from build123d import *

# Parameters (mm, degrees)
BOSS_EXTRUDE1_DEPTH              = 3.175
F_6_CLEARANCE_HOLE1_D            = 4.3053
F_6_CLEARANCE_HOLE2_D            = 4.3053
F_9_64_0_14063_DIAMETER_HOLE1_D  = 3.572002
F_15_32_0_46875_DIAMETER_HOLE1_D = 11.90625
F_1_2_0_5_DIAMETER_HOLE1_D       = 12.7
CUT_EXTRUDE1_REACH               = 5.175
SKETCH12_W                       = 9.525
SKETCH12_H                       = 31.75
FILLET1_R                        = 9.525


with BuildPart() as part:
    # Sketch1 → Boss-Extrude1 (new body)
    with BuildSketch(Plane.XY):
        with BuildLine():
            Line((-29.21, 1.5875), (-29.21, 0))
            Line((-29.21, 0), (0, 0))
            Line((0, 0), (0, 165.1))
            Line((0, 165.1), (-25.4, 165.1))
            Line((-25.4, 165.1), (-25.4, 138.1125))
            ThreePointArc((-25.4, 138.1125), (-26.794903955, 134.744903955), (-30.1625, 133.35))
            Line((-30.1625, 133.35), (-53.848, 133.35))
            Line((-53.848, 133.35), (-59.411809524, 6.35))
            Line((-59.411809524, 6.35), (-33.9725, 6.35))
            ThreePointArc((-33.9725, 6.35), (-30.604903955, 4.955096045), (-29.21, 1.5875))
        make_face()
    extrude(amount=-BOSS_EXTRUDE1_DEPTH)

    # #6 Clearance Hole1 (through all)
    with Locations(Plane.XY):
        with Locations((-47.625, 128.5875), (-6.35, 149.86), (-50.546, 16.51), (-6.35, 16.51)):
            Hole(F_6_CLEARANCE_HOLE1_D / 2)

    # #6 Clearance Hole2 (through all)
    with Locations(Plane.XY):
        with Locations((-43.18, 37.084), (-20.32, 120.65)):
            Hole(F_6_CLEARANCE_HOLE2_D / 2)

    # 9/64 (0.14063) Diameter Hole1 (through all)
    with Locations(Plane.XY):
        with Locations((-38.1, 98.425), (-36.5125, 30.1625)):
            Hole(F_9_64_0_14063_DIAMETER_HOLE1_D / 2)

    # 15/32 (0.46875) Diameter Hole1 (through all)
    with Locations(Plane.XY):
        with Locations((-11.684, 88.9)):
            Hole(F_15_32_0_46875_DIAMETER_HOLE1_D / 2)

    # 1/2 (0.5) Diameter Hole1 (through all)
    with Locations(Plane.XY):
        with Locations((-38.1, 88.9), (-26.9875, 30.1625)):
            Hole(F_1_2_0_5_DIAMETER_HOLE1_D / 2)

    # Sketch12 → Cut-Extrude1 (cut, up to next)
    with BuildSketch(Plane.XY, mode=Mode.PRIVATE) as cut_extrude1_sk1:
        with Locations((-25.4, 149.225)):
            Rectangle(SKETCH12_W, SKETCH12_H)
    cut_extrude1_tool1 = extrude(cut_extrude1_sk1.sketch, amount=-CUT_EXTRUDE1_REACH, mode=Mode.PRIVATE) & part.part
    add(cut_extrude1_tool1.solids().sort_by_distance((-25.4, 149.225, 0))[0], mode=Mode.SUBTRACT)

    # Fillet1
    fillet1_edges = [part.edges().sort_by_distance(p)[0] for p in [
        (-20.6375, 133.35, -1.5875),
    ]]
    fillet(fillet1_edges, radius=FILLET1_R)


solid = part.part
Design review of the part built by this model. Coordinates are the model's own, in mm. A direction names the side the tool comes from. Round coordinates to 2 decimals unless told otherwise and drop trailing zeros. Loops run counter-clockwise (first coordinate to the right, second up) from the corner with the lowest first, then second, coordinate; pieces in that order, holes last. Notation, with made-up numbers: (32, 55.5) -> (51, 55.5) arc R29 cw to (51, 77.5) -> close; hole circle Ø10 at (24, 25). An arc over 180 degrees is marked (long way). Use one line per item in the form item = value. Start each with the question number.
Q1. We need section C-C on y = 16.51. Give the boundary of the cut face in (x, z) (3 decimals).
Q2. Draft analysis for pull direction Y (two halves, no side actions). For faces 1 (the face through (-35.196, 31.37, -1.61)), 2 (the face through (-37.713, 96.681, -1.61)), 3 (the face through (-10, 165.1, -2)), 4 (the face through (-20.638, 154, -2)), state which applies: +Y half, -Y half, draft (parallel to the pull), parting line (faces both ways), or undercut.
Q3. For pin 1 Ø1.6 at (x, z) = (-48, -1.5) entering from -Y; pin 2 Ø1.6 at (x, z) = (-40, -1) entering from +Y; pin 3 Ø1.5 at (y, z) = (75, -1) entering from -X, all flat-tipped, find the tip position at first contact; note any pin that passes through.
Q4. Wall thickness on line 1 along Y through (x, z) = (-47.5, -0.55); line 2 along Y through (x, z) = (-43.18, -1.15); line 3 along Y through (x, z) = (-38, -1.2): over which ranges is each line inside the solid? List them lowest first. Write a range as [from, to].
Q5. We need section B-B on x = -24. Give the boundary of the cut face in (y, z) (3 decimals), then the cut area to 3 significant figures.
Q6. Machinability: for faces 5 (the face through (-15, 0, -2)), 6 (the face through (-47, 6.35, -2)), which of the approach directions +Z, -Z, +X, -X, +Y, -Y give a long, thin tool a straight path to every point of the face, cutting with its end or side? Answer none if there is none.
Q7. We need section D-D on z = -2.2. State how many separate pieces and enclosed holes the cut face has, then the cut area to 4 significant figures.
Q8. We need section A-A on y = 120.65. Give the boundary of the cut face in (x, z) (3 decimals).
Calculated:
q1.outline = (-58.967, -3.175) -> (-52.699, -3.175) -> (-52.699, 0) -> (-58.967, 0) -> close; (-48.393, -3.175) -> (-8.503, -3.175) -> (-8.503, 0) -> (-48.393, 0) -> close; (-4.197, -3.175) -> (0, -3.175) -> (0, 0) -> (-4.197, 0) -> close
q2.face_1 = undercut
q2.face_2 = undercut
q2.face_3 = +Y half
q2.face_4 = draft
q3.pin_1 = 6.35
q3.pin_2 = 133.35
q3.pin_3 = -56.44
q4.line_1 = [6.35, 126.44], [130.74, 133.35]
q4.line_2 = [6.35, 34.93], [39.24, 85.09], [92.71, 133.35]
q4.line_3 = [6.35, 29.17], [31.15, 82.55], [95.25, 96.64], [100.21, 133.35]
q5.outline = (0, -3.175) -> (24.559, -3.175) -> (24.559, 0) -> (0, 0) -> close; (35.766, -3.175) -> (135.612, -3.175) -> (135.612, 0) -> (35.766, 0) -> close
q5.area = 395 mm²
q6.face_5 = +Z, -Z, +X, -X, -Y
q6.face_6 = +Z, -Z, -X, -Y
q7.separate_pieces = 1
q7.enclosed_holes = 11
q7.area = 7,585 mm²
q8.outline = (-54.404, -3.175) -> (-22.473, -3.175) -> (-22.473, 0) -> (-54.404, 0) -> close; (-18.167, -3.175) -> (0, -3.175) -> (0, 0) -> (-18.167, 0) -> close
